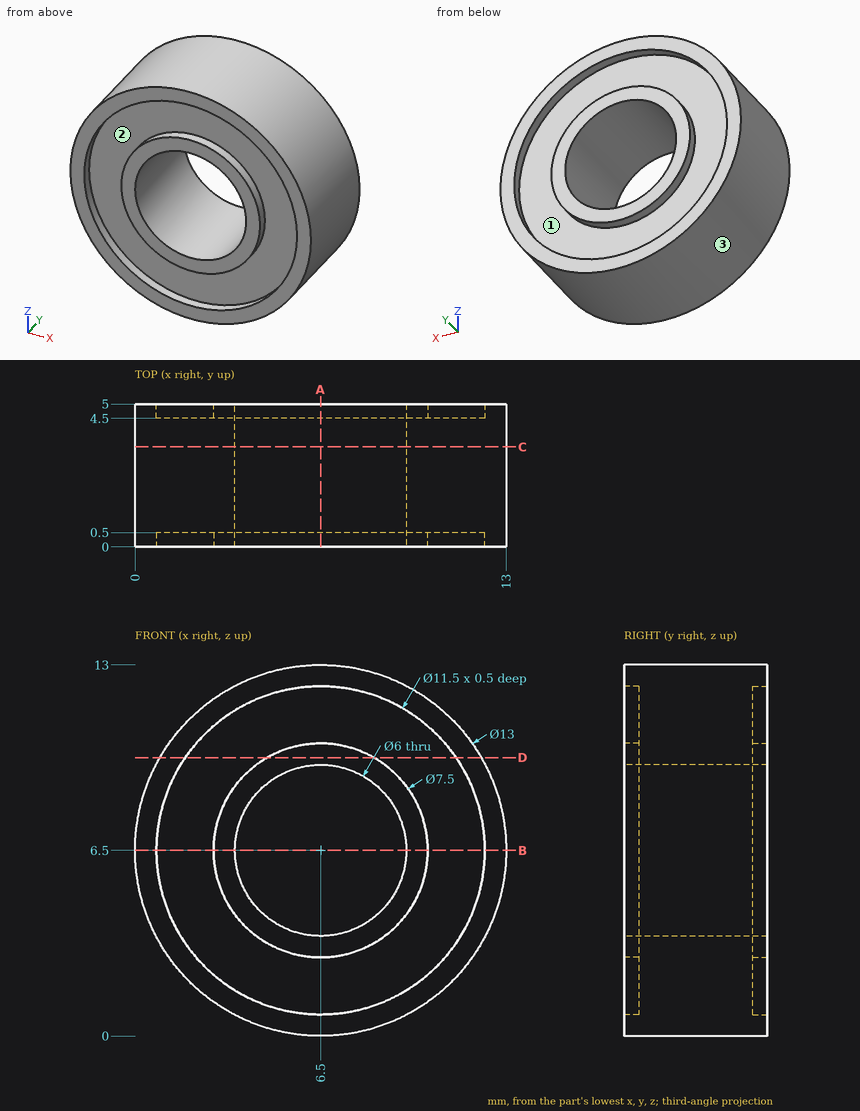
Geometry check sheet. Reference: drawing and pictorial views, mm from the part's lowest x, y, z. A direction names the side the tool comes from. Coordinates: 2 decimals unless noted, no trailing zeros. Loops run counter-clockwise (first coordinate to the right, second up) from the corner with the lowest first, then second, coordinate; pieces in that order, holes last. Notation, with made-up numbers: (4.25, 30.5) - (52.25, 30.5) arc R23 cw to (52.25, 67.5) - close; hole circle Ø2 at (28.25, 42). An arc over 180 degrees is marked (long way). Return JSON: item names as keys, results as strings.
1. Section check D-D, the plane z = 9.75. Record the boundary of the cut face in (x, y).
Established:
{"outline": "(0.87, 0) - (1.76, 0) - (1.76, 0.5) - (4.63, 0.5) - (4.63, 0) - (8.37, 0) - (8.37, 0.5) - (11.24, 0.5) - (11.24, 0) - (12.13, 0) - (12.13, 5) - (11.24, 5) - (11.24, 4.5) - (8.37, 4.5) - (8.37, 5) - (4.63, 5) - (4.63, 4.5) - (1.76, 4.5) - (1.76, 5) - (0.87, 5) - close"}
2. Tool access check on the marked faces 1, 2 and 3. Record the directions out of +Z, -Z, +X, -X, +Y, -Y that give a thin tool (end or side, any length) a straight path to the whole face; none if there is none.
Established:
{"face 1": "+Y", "face 2": "-Y", "face 3": "+Y, -Y"}
3. Thickness scan on L1, parallel to Z at x = 6.5, y = 0.1; L2, parallel to Z at x = 6.5, y = 1.5; L3, parallel to Y at x = 11.25, z = 6.5. Record the ranges inside material, lowest first.
Established:
{"L1": "z = 0 to 0.75, 2.75 to 3.5, 9.5 to 10.25, 12.25 to 13", "L2": "z = 0 to 3.5, 9.5 to 13", "L3": "y = 0.5 to 4.5"}
4. Section check C-C, the plane y = 3.5. Record the boundary of the cut face in (x, z).
Established:
{"outline": "circle Ø13 at (6.5, 6.5); hole circle Ø6 at (6.5, 6.5)"}
5. Section check B-B, the plane z = 6.5. Record the boundary of the cut face in (x, y), then the cut area to 3 significant figures.
Established:
{"outline": "(0, 0) - (0.75, 0) - (0.75, 0.5) - (2.75, 0.5) - (2.75, 0) - (3.5, 0) - (3.5, 5) - (2.75, 5) - (2.75, 4.5) - (0.75, 4.5) - (0.75, 5) - (0, 5) - close; (9.5, 0) - (10.25, 0) - (10.25, 0.5) - (12.25, 0.5) - (12.25, 0) - (13, 0) - (13, 5) - (12.25, 5) - (12.25, 4.5) - (10.25, 4.5) - (10.25, 5) - (9.5, 5) - close", "area": "31.0 mm2"}
6. Section check A-A, the plane x = 6.5. Record the boundary of the cut face in (y, z), then the cut area to 3 significant figures.
Established:
{"outline": "(0, 0) - (5, 0) - (5, 0.75) - (4.5, 0.75) - (4.5, 2.75) - (5, 2.75) - (5, 3.5) - (0, 3.5) - (0, 2.75) - (0.5, 2.75) - (0.5, 0.75) - (0, 0.75) - close; (0, 9.5) - (5, 9.5) - (5, 10.25) - (4.5, 10.25) - (4.5, 12.25) - (5, 12.25) - (5, 13) - (0, 13) - (0, 12.25) - (0.5, 12.25) - (0.5, 10.25) - (0, 10.25) - close", "area": "31.0 mm2"}
7. Go/stop test with flat-tipped pins: pin 1 (3 mm diameter, centred on x = 2.5, y = 2, fed in from -Z); pin 2 (3 mm diameter, centred on y = 1.5, z = 9.5, fed in from -X); pin 3 (1 mm diameter, centred on x = 3, y = 2.5, fed in from +Z). Record where each tip stops, or that it passes through.
Established:
{"pin 1": "stops at z = 0.5", "pin 2": "stops at x = 0.18", "pin 3": "stops at z = 12.27"}
